The listing builds one solid part. Answer for the finished solid, in the listing's coordinates (mm). A direction names the side the tool comes from. Give positions to 0.01 mm unless a question says otherwise; leave off trailing zeros. Write each loop counter-clockwise with the first axis right and the second up, starting at its lowest first coordinate (ties: lowest second). Pieces come first, ordered by that corner, then holes. Notation, with made-up numbers: (-14.75, 18) -> (7.25, 18) arc R22 cw to (7.25, 50) -> close; hole circle Ø1 at (88.5, 62). An arc over 180 degrees is marked (long way). One line per question, with ' | ' between items.
from build123d import *

# Parameters (mm, degrees)
SKETCH_1_R          = 1.875
SKETCH_1_R_2        = 1.25
EXTRUDE_1_DEPTH     = 5
FILLET_1_R          = 3
FILLET_2_R          = 5
FILLET_3_R          = 3
SKETCH_2_R          = 3.15
CUT_EXTRUDE_1_DEPTH = 4
SKETCH_3_R          = 2
CUT_EXTRUDE_2_DEPTH = 79.665430781


with BuildPart() as part:
    # Эскиз1 → Бобышка-Вытянуть1 (new body)
    with BuildSketch(Plane.XY):
        with BuildLine():
            Line((0, 0), (20, 0))
            Line((20, 0), (25.5, 6.006432896))
            Line((25.5, 6.006432896), (45.5, 6.006432896))
            Line((45.5, 6.006432896), (51, 0))
            Line((51, 0), (71, 0))
            Line((71, 0), (71, 28))
            Line((71, 28), (49.07387196, 28))
            ThreePointArc((49.07387196, 28), (35.5, 33.5), (21.92612804, 28))
            Line((21.92612804, 28), (0, 28))
            Line((0, 28), (0, 0))
        make_face()
        with Locations((35.5, 30.25)):
            Circle(SKETCH_1_R, mode=Mode.SUBTRACT)
        with Locations((35.5, 14)):
            Circle(SKETCH_1_R_2, mode=Mode.SUBTRACT)
        with Locations((49.572912812, 5.875)):
            Circle(SKETCH_1_R, mode=Mode.SUBTRACT)
        with Locations((21.427087189, 5.875)):
            Circle(SKETCH_1_R, mode=Mode.SUBTRACT)
    extrude(amount=EXTRUDE_1_DEPTH)

    # Скругление1
    fillet_1_edges = [part.edges().sort_by_distance(p)[0] for p in [
        (21.92612804, 28, 2.5),
        (49.07387196, 28, 2.5),
        (45.5, 6.006432896, 2.5),
        (25.5, 6.006432896, 2.5),
    ]]
    fillet(fillet_1_edges, radius=FILLET_1_R)

    # Скругление2
    fillet_2_edges = [part.edges().sort_by_distance(p)[0] for p in [
        (0, 28, 2.5),
        (71, 28, 2.5),
        (71, 0, 2.5),
        (0, 0, 2.5),
    ]]
    fillet(fillet_2_edges, radius=FILLET_2_R)

    # Скругление3
    fillet_3_edges = [part.edges().sort_by_distance(p)[0] for p in [
        (51, 0, 2.5),
        (20, 0, 2.5),
    ]]
    fillet(fillet_3_edges, radius=FILLET_3_R)

    # Эскиз2 → Вырез-Вытянуть1 (cut)
    with BuildSketch(Plane.XY.offset(5)):
        with Locations((35.5, 14)):
            Circle(SKETCH_2_R)
    extrude(amount=-CUT_EXTRUDE_1_DEPTH, mode=Mode.SUBTRACT)

    # Эскиз3 → Вырез-Вытянуть2 (cut, through all)
    with BuildSketch(Plane(origin=(0, 0, 0), x_dir=(-1, 0, 0), z_dir=(0, 0, -1))):
        with Locations((-10.5, 14)):
            Circle(SKETCH_3_R)
        with Locations((-60.5, 14)):
            Circle(SKETCH_3_R)
    extrude(amount=-CUT_EXTRUDE_2_DEPTH, mode=Mode.SUBTRACT)


solid = part.part
Item 1: Consider line 1 (Y direction, x = 60.5, z = 1.55); line 2 (X direction, y = 15.5, z = 1.95); line 3 (X direction, y = 4.5, z = 1.9). Determine where each line is inside the solid, lowest interval first. Write a range as [from, to].
Answers below:
line 1: [0, 12], [16, 28] | line 2: [0, 9.18], [11.82, 32.73], [38.27, 59.18], [61.82, 71] | line 3: [0.03, 20.15], [22.7, 24.12], [46.88, 48.3], [50.85, 70.97]
Item 2: Find section C-C (z = 2.4). Write down the section's boundary in (x, y) (3 decimals), then the cut area to 3 significant figures.
Answers below:
outline: (0, 5) arc R5 ccw to (5, 0) -> (18.679, 0) arc R3 ccw to (20.892, 0.974) -> (24.608, 5.032) arc R3 cw to (26.821, 6.006) -> (44.179, 6.006) arc R3 cw to (46.392, 5.032) -> (50.108, 0.974) arc R3 ccw to (52.321, 0) -> (66, 0) arc R5 ccw to (71, 5) -> (71, 23) arc R5 ccw to (66, 28) -> (50.239, 28) arc R3 cw to (48.274, 28.733) arc R19.5 ccw to (22.726, 28.733) arc R3 cw to (20.761, 28) -> (5, 28) arc R5 ccw to (0, 23) -> close; hole circle Ø4 at (10.5, 14); hole circle Ø3.75 at (21.427, 5.875); hole circle Ø6.3 at (35.5, 14); hole circle Ø3.75 at (35.5, 30.25); hole circle Ø3.75 at (49.573, 5.875); hole circle Ø4 at (60.5, 14) | area: 1,830 mm²
Item 3: Determine the mould class of faces 4 (the face through (11.974, 15.352, 2.465)), 5 (the face through (69, 1, 3)), 6 (the face through (35.7, 33.5, 2.5)), 7 (the face through (35, 21, 5)) for opening direction X: pulls with the +X half, pulls with the -X half, needs draft (parallel to the pull), parting line crosses it, or undercut.
Answers below:
face 4: undercut | face 5: pulls with the +X half | face 6: parting line crosses it | face 7: needs draft
Item 4: Find section A-A (x = 35.5). Write down the section's boundary in (y, z) (3 decimals), then the cut area to 3 significant figures.
Answers below:
outline: (6.006, 0) -> (12.75, 0) -> (12.75, 1) -> (10.85, 1) -> (10.85, 5) -> (6.006, 5) -> close; (15.25, 0) -> (28.375, 0) -> (28.375, 5) -> (17.15, 5) -> (17.15, 1) -> (15.25, 1) -> close; (32.125, 0) -> (33.5, 0) -> (33.5, 5) -> (32.125, 5) -> close | area: 91.0 mm²
Item 5: Find section D-D (y = 3). Write down the section's boundary in (x, z).
Answers below:
outline: (0.42, 0) -> (22.75, 0) -> (22.75, 5) -> (0.42, 5) -> close; (48.25, 0) -> (70.58, 0) -> (70.58, 5) -> (48.25, 5) -> close
Item 6: A tool of negligible diameter and unlimited length cuts with its end or side. For faces 1 (the face through (37, 14, 1)), 2 (the face through (45.37, 5.76, 2.54)), 3 (the face through (13, 28, 2)), from which of +Z, -Z, +X, -X, +Y, -Y can it reach the whole face along a straight path? Write none if from no direction.
Answers below:
face 1: +Z | face 2: +Z, -Z, -Y | face 3: +Z, -Z, -X, +Y
Item 7: Flat-ended cylindrical pins translate along their axes: pin 1 (1.9 mm diameter, centred on x = 37, y = 13.5, fed in from +Z); pin 2 (1.5 mm diameter, centred on x = 10.5, z = 3.5, fed in from +Y). Find the tip coordinate at first contact, or state that the pin passes through.
Answers below:
pin 1: z = 1 | pin 2: y = 28
Item 8: Find section B-B (x = 60.5). Write down the section's boundary in (y, z), then the cut area to 3 significant figures.
Answers below:
outline: (0, 0) -> (12, 0) -> (12, 5) -> (0, 5) -> close; (16, 0) -> (28, 0) -> (28, 5) -> (16, 5) -> close | area: 120 mm²
